Work out the finished part from the listing and answer in its coordinate system (mm). A direction names the side the tool comes from. Coordinates: 2 decimals unless noted, no trailing zeros. Write each loop counter-clockwise with the first axis right and the second up, starting at its lowest first coordinate (ties: lowest second). Pieces come first, ordered by that corner, then holes. Notation, with made-up numbers: (-9.5, -21.75) - (4.5, -21.75) arc R13 ccw to (4.5, -10.75) - close; hole circle Ø3 at (-7.5, -19.75). An arc over 180 degrees is marked (long way). Use a Markdown table: item, result. Add a question column.
(1) For a pull along X with two mould halves and no side action, classify faces 6 (the face through (1.8, -1.6, 5)), 7 (the face through (5.6, -0.02, -1.21)), 8 (the face through (4.4, 0, 1.5)) as released by +X, released by -X, zero draft, split by the parting line, or undercut.
(2) The part is cut by section A-A, the plane x = 0. Give the vertices of the cut face in (y, z).
(3) Given pin 1 Ø0.5 at (x, y) = (4.5, -0.5) entering from -Z; pin 2 Ø2 at (y, z) = (2, 1) entering from -X; pin 3 Ø0.6 at (x, z) = (4.5, 0) entering from -Y; pin 4 Ø2 at (x, z) = (-1.5, -3) entering from +Y, each flat-ended and moving along its own axis, determine where each tip first touches the part or whether it passes through.
(4) Find the intervals of material crossed by line 1 (X direction, y = 0.7, z = 0); line 2 (X direction, y = -5.5, z = 2); line 3 (Z direction, x = 4.5, y = 1.25), in increasing order. Write a range as from..to.
(5) The part is cut by section B-B, the plane x = -1.75. Give the vertices of the cut face in (y, z), then the cut area to 3 significant figures.
(6) A tool of negligible diameter and unlimited length cuts with its end or side. For faces 1 (the face through (1.148, -4, -4)), 2 (the face through (5.1, -1.5, 0)), 3 (the face through (4.4, 0, -1.5)), 4 (the face through (-3.28, 0.91, 0.47)), 5 (the face through (5.1, 1.5, 0)), from which of +Z, -Z, +X, -X, +Y, -Y can it reach the whole face along a straight path? Write none if from no direction.
Autodesk Inventor part; units mm, degrees
ref_plane "YZ Plane" through (0, 0, 0) normal (1, 0, 0) x (0, 1, 0)
ref_plane "XZ Plane" through (0, 0, 0) normal (0, 1, 0) x (-1, 0, 0)
ref_plane "XY Plane" through (0, 0, 0) normal (0, 0, 1) x (1, 0, 0)
sketch "Sketch1" plane through (0, 0, 0) normal (0, 1, 0) x (-1, 0, 0)
  line L0 (3.8975, 0) -> (0.3525, 5.9)
  line L1 (0.3525, 5.9) -> (-1.1475, 5.9)
  line L2 (-1.1475, 5.9) -> (-1.1475, 5.25)
  line L3 (-1.1475, 5.25) -> (-2.3975, 5.25)
  line L4 (-2.3975, 5.25) -> (-2.3975, 5.9)
  line L5 (-2.3975, 5.9) -> (-3.8975, 5.9)
  line L6 (-3.8975, 5.9) -> (-3.8975, 0)
  line L7 (-3.8975, 0) -> (3.8975, 0)
  point P0 (0, 0)
  point P1 (0, 0)
  dimension "d0" = 11.8
  dimension "d1" = 1.25
  dimension "d2" = 10.5
  dimension "d3" = 59
  dimension "d4" = 1.5
revolve "Revolution1" add sketch "Sketch1" angle 360 about axis through (3.8975, 0, 0) along (-1, 0, 0)
sketch "Sketch2" plane through (3.8975, 0, 0) normal (1, 0, 0) x (0, 0, -1)
  line L0 (1.5, -1.5) -> (-1.5, -1.5)
  line L1 (-1.5, -1.5) -> (-1.5, 1.5)
  line L2 (-1.5, 1.5) -> (1.5, 1.5)
  line L3 (1.5, 1.5) -> (1.5, -1.5)
  line L4 (1.5, -1.5) -> (-1.5, 1.5) construction
  line L5 (-1.5, -1.5) -> (1.5, 1.5) construction
  point P0 (0, 0)
  dimension "d6" = 3
  dimension "d7" = 3
extrude "Extrusion1" add sketch "Sketch2" along normal blind 2
sketch "Sketch3" plane through (3.8975, -1.5, -1.5) normal (0, -1, 0) x (1, 0, 0)
  line L0 (0, 0) -> (0, 3)
  line L1 (0, 0) -> (2, 0)
  line L2 (2, 3) -> (2, 0)
  line L3 (0, 3) -> (2, 3)
  circle A0 centre (0.5, 1.5) radius 0.5
  line L4 (0, 7.4) -> (0, -4.4)
  point P0 (-3.8975, 1.5)
  dimension "d10" = 1
extrude "Extrusion2" cut sketch "Sketch3" against normal through all contours A0
fillet "Fillet1" radius 1 2 edges at (5.8975, 0, 1.5) (5.8975, 0, -1.5)
properties part number "PayloadGermination_SyringePlunger" material "Aluminum 6061"
Model answer:
| question | item | result |
|---|---|---|
| 1 | face 6 | undercut |
| 1 | face 7 | released by +X |
| 1 | face 8 | zero draft |
| 2 | outline | circle Ø11.8 at (0, 0) |
| 3 | pin 1 | z = -1.5 |
| 3 | pin 2 | x = -3.15 |
| 3 | pin 3 | through |
| 3 | pin 4 | y = 4.88 |
| 4 | line 1 | -3.48..3.9, 4.9..5.9 |
| 4 | line 2 | -0.38..1.15, 2.4..3.9 |
| 4 | line 3 | -1.5..-0.49, 0.49..1.5 |
| 5 | outline | circle Ø7.15 at (0, 0) |
| 5 | area | 40.1 mm^2 |
| 6 | face 1 | none |
| 6 | face 2 | +Z, -Z, +X, -Y |
| 6 | face 3 | -Z, +X, +Y, -Y |
| 6 | face 4 | -X |
| 6 | face 5 | +Z, -Z, +X, +Y |
